Geometry: final body of the model. Coordinates: model frame, mm. Face numbers are marked on the shaded views. A direction names the side the tool comes from. Round coordinates to 2 decimals unless told otherwise and drop trailing zeros. Loops run counter-clockwise (first coordinate to the right, second up) from the corner with the lowest first, then second, coordinate; pieces in that order, holes last. Notation, with made-up numbers: (19.25, 22) -> (28.25, 22) arc R22 ccw to (28.25, 49) -> close; hole circle Ø2 at (-7.75, -29). An arc over 180 degrees is marked (long way). Answer in a Markdown table with one row per item.
```python
from build123d import *

# Parameters (mm, degrees)
SKETCH1_R           = 13
SKETCH1_R_2         = 8
BOSS_EXTRUDE1_DEPTH = 5
CUT_EXTRUDE1_START  = -5
CUT_EXTRUDE1_DEPTH  = 3
CUT_EXTRUDE2_START  = 2
CUT_EXTRUDE2_DEPTH  = 3


with BuildPart() as part:
    # Sketch1 → Boss-Extrude1 (new, symmetric)
    with BuildSketch(Plane(origin=(0, 0, 0), x_dir=(1, 0, 0), z_dir=(0, 1, 0))):
        with BuildLine():
            Line((22.5, 0), (12.5, 130))
            ThreePointArc((12.5, 130), (0, 142.5), (-12.5, 130))
            Line((-12.5, 130), (-22.5, 0))
            ThreePointArc((-22.5, 0), (0, -22.5), (22.5, 0))
        make_face()
        with Locations(Location((0, 0, 0), (0, 0, 270))):
            Circle(SKETCH1_R, mode=Mode.SUBTRACT)
        with Locations(Location((0, 130, 0), (0, 0, 270))):
            Circle(SKETCH1_R_2, mode=Mode.SUBTRACT)
    extrude(amount=BOSS_EXTRUDE1_DEPTH, both=True)

    # Sketch2 → Cut-Extrude1 (cut)
    with BuildSketch(Plane(origin=(0, 0, 0), x_dir=(1, 0, 0), z_dir=(0, 1, 0)).offset(CUT_EXTRUDE1_START)):
        with BuildLine():
            Line((-8.210272961, 120.57442745), (-17.265674906, 2.854202174))
            ThreePointArc((-17.265674906, 2.854202174), (0, 17.5), (17.265674906, 2.854202174))
            Line((17.265674906, 2.854202174), (8.210272961, 120.57442745))
            ThreePointArc((8.210272961, 120.57442745), (0, 117.5), (-8.210272961, 120.57442745))
        make_face()
    extrude(amount=CUT_EXTRUDE1_DEPTH, mode=Mode.SUBTRACT)

    # Sketch2<3> → Cut-Extrude2 (cut)
    with BuildSketch(Plane(origin=(0, 0, 0), x_dir=(1, 0, 0), z_dir=(0, 1, 0)).offset(CUT_EXTRUDE2_START)):
        with BuildLine():
            Line((-8.210272961, 120.57442745), (-17.265674906, 2.854202174))
            ThreePointArc((-17.265674906, 2.854202174), (0, 17.5), (17.265674906, 2.854202174))
            Line((17.265674906, 2.854202174), (8.210272961, 120.57442745))
            ThreePointArc((8.210272961, 120.57442745), (0, 117.5), (-8.210272961, 120.57442745))
        make_face()
    extrude(amount=CUT_EXTRUDE2_DEPTH, mode=Mode.SUBTRACT)


solid = part.part
```
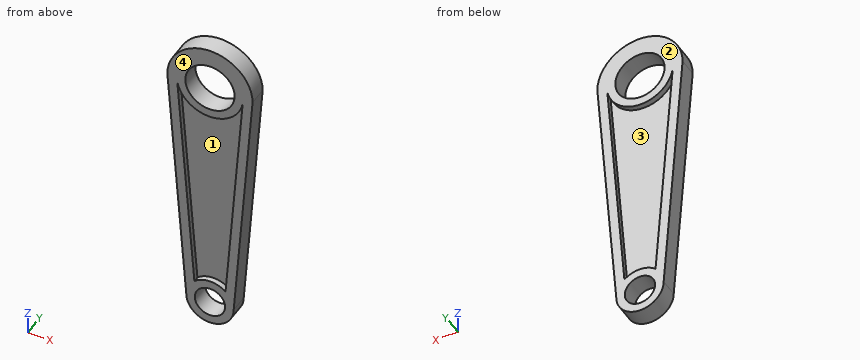
Item 1: Section query C-C, the plane x = -11. Output: boundary loops of the cut face in (y, z), and give its area (3 significant figures).
Ans:
| item | result |
|---|---|
| outline | (-5, -135.94) -> (5, -135.94) -> (5, -84.31) -> (2, -84.31) -> (2, -13.61) -> (5, -13.61) -> (5, -6.93) -> (-5, -6.93) -> (-5, -13.61) -> (-2, -13.61) -> (-2, -84.31) -> (-5, -84.31) -> close; (-5, 6.93) -> (5, 6.93) -> (5, 19.63) -> (-5, 19.63) -> close |
| area | 993 mm2 |
Item 2: Set-up query: the marked faces 3 and 4. Return all of +Z, -Z, +X, -X, +Y, -Y with unobstructed straight access to the full face (end or side cutting, diameter ignored); none if empty.
Ans:
| item | result |
|---|---|
| face 3 | +Y |
| face 4 | +Z, -Z, +X, -X, -Y |
Item 3: Section query B-B, the plane y = -3.5. Output: boundary loops of the cut face in (x, z).
Ans:
| item | result |
|---|---|
| outline | (-22.5, 0) -> (-12.5, -130) arc R12.5 ccw to (12.5, -130) -> (22.5, 0) arc R22.5 ccw to start; hole (-17.27, -2.85) -> (-8.21, -120.57) arc R12.5 cw to (8.21, -120.57) -> (17.27, -2.85) arc R17.5 cw to start; hole circle Ø26 at (0, 0); hole circle Ø16 at (0, -130) |
Item 4: Ray query, L1, parallel to Z at x = 0.5, y = -1.5; L2, parallel to X at y = -0.5, z = -130; L3, parallel to Z at x = 6.5, y = 3.75. Return the intervals inside material, ascending.
Ans:
| item | result |
|---|---|
| L1 | -142.49 to -137.98, -122.02 to -12.99, 12.99 to 22.49 |
| L2 | -12.5 to -8, 8 to 12.5 |
| L3 | -140.68 to -134.66, -125.34 to -119.32, -16.25 to -11.26, 11.26 to 21.54 |
Item 5: First-contact query: P1, Ø4, axis at x = 8.5, y = -0.5, coming from the +Z side; P2, Ø5, axis at y = 2.5, z = -23.5, coming from the -X side; P3, Ø5, axis at x = -17.5, y = -1, coming from the +Z side. Flat tips, straight axial feed; report the tip coordinate or a pass-through.
Ans:
| item | result |
|---|---|
| P1 | z = 21.54 |
| P2 | x = -20.88 |
| P3 | z = 16.77 |
Item 6: Mould query, pull axis Z, two halves, no side actions, for the marked faces 1 and 2. Classes: released by +Z, released by -Z, zero draft, split by the parting line, or undercut.
Ans:
| item | result |
|---|---|
| face 1 | undercut |
| face 2 | zero draft |
Item 7: Section query D-D, the plane z = -109.5. Output: boundary loops of the cut face in (x, y).
Ans:
| item | result |
|---|---|
| outline | (-14.08, -5) -> (-9.06, -5) -> (-9.06, -2) -> (9.06, -2) -> (9.06, -5) -> (14.08, -5) -> (14.08, 5) -> (9.06, 5) -> (9.06, 2) -> (-9.06, 2) -> (-9.06, 5) -> (-14.08, 5) -> close |
Item 8: Section query A-A, the plane x = 0. Output: boundary loops of the cut face in (y, z).
Ans:
| item | result |
|---|---|
| outline | (-5, -142.5) -> (5, -142.5) -> (5, -138) -> (-5, -138) -> close; (-5, -122) -> (5, -122) -> (5, -117.5) -> (2, -117.5) -> (2, -17.5) -> (5, -17.5) -> (5, -13) -> (-5, -13) -> (-5, -17.5) -> (-2, -17.5) -> (-2, -117.5) -> (-5, -117.5) -> close; (-5, 13) -> (5, 13) -> (5, 22.5) -> (-5, 22.5) -> close |
